Autodesk Inventor part; units mm, degrees
ref_plane "YZ Plane" through (0, 0, 0) normal (1, 0, 0) x (0, 1, 0)
ref_plane "XZ Plane" through (0, 0, 0) normal (0, 1, 0) x (-1, 0, 0)
ref_plane "XY Plane" through (0, 0, 0) normal (0, 0, 1) x (1, 0, 0)
sketch "スケッチ1" plane through (0, 0, 0) normal (0, 0, 1) x (1, 0, 0)
  circle A0 centre (0, 0) radius 1.65
  dimension "d0" = 3.3
extrude "押し出し1" add sketch "スケッチ1" along normal blind 25
sketch "スケッチ2" plane through (0, 0, 25) normal (0, 0, 1) x (1, 0, 0)
  circle A0 centre (0, 0) radius 4
  dimension "d3" = 8
extrude "押し出し2" add sketch "スケッチ2" against normal blind 2.3
chamfer "面取り1" distance 2.3 angle 45 1 edges at (-4, 0, 22.7)
thread "ねじ1"
properties part number "ネジ皿m4,25" material "鋼、高強度、低合金"
Could you check a few things on this model? Use its own coordinates, in mm. A direction names the side the tool comes from. Give positions to 0.01 mm unless a question says otherwise; leave off trailing zeros. Order: outer loops, then holes, each group sorted by start corner. A loop starts at its lowest first (then second) coordinate and runs counter-clockwise, first axis right, second up.
Q1. Suppose I cut it at C-C, the plane z = 14.75. Write out the boundary of the cut face in (x, y).
Q2. If I drill on line 1 along X through (y, z) = (0, 3.25); line 2 along Y through (x, z) = (0.75, 11); line 3 along Y through (x, z) = (-0.5, 9.5), over which ranges is the centre line in solid material (lowest first)?
Q3. For faces 1 (the cylindrical face through (-1.216, -1.115, 11.191)), 2 (the flat face through (0, 0, 25)), which set-ups out of +Z, -Z, +X, -X, +Y, -Y let a thin tool reach every point of the face, with its end or its side?
Q4. I'm going to push flat-ended pins straight in: P1, Ø3, axis at y = -1.5, z = 4.5, coming from the +X side; P2, Ø2, axis at x = -1, z = 7, coming from the -Y side; P3, Ø1.5, axis at x = -2.5, y = 0, coming from the -Z side. Where does each tip first touch, or does it pass through?
Solution:
1. outline: circle Ø3.3 at (0, 0)
2. line 1: x = -1.65 to 1.65
2. line 2: y = -1.47 to 1.47
2. line 3: y = -1.57 to 1.57
3. face 1: -Z
3. face 2: +Z, +X, -X, +Y, -Y
4. P1: stops at x = 1.65
4. P2: stops at y = -1.65
4. P3: stops at z = 22.75
